Input: part model. Units: mm. Frame: model coordinates. A direction names the side the tool comes from. Give positions to 0.01 mm unless a question says otherwise; leave off trailing zeros. Loops run counter-clockwise (first coordinate to the right, second up) from the corner with the lowest first, then second, coordinate; pieces in that order, holes last. Notation, with made-up numbers: (49, 17.25) - (106, 17.25) arc R17 cw to (106, 29.25) - close; hole circle Ø9 at (51, 61). An arc over 180 degrees is marked (long way). Answer as a JSON object with one key per item and string values.
Autodesk Inventor part; units mm, degrees
ref_plane "Work Plane1" through (31.75, 0, 0) normal (1, 0, 0) x (0, 1, 0)
ref_plane "XZ Plane" through (0, 0, 0) normal (0, 1, 0) x (-1, 0, 0)
ref_plane "XY Plane" through (0, 0, 0) normal (0, 0, 1) x (1, 0, 0)
sketch "Sketch1" plane through (0, 0, 0) normal (0, 1, 0) x (-1, 0, 0)
  circle A0 centre (0, 0) radius 25.4
  circle A1 centre (0, 0) radius 31.75
  dimension "d0" = 50.8
  dimension "d1" = 63.5
extrude "Extrusion1" add sketch "Sketch1" along normal blind 6.35
sketch "Sketch2" plane through (0, 0, 0) normal (0, -1, 0) x (1, 0, 0)
  circle A0 centre (0, 0) radius 25.654
  circle A1 centre (0, 0) radius 31.75
  dimension "d4" = 51.308
extrude "Extrusion2" add sketch "Sketch2" along normal blind 25.4
chamfer "Chamfer1" distance 3.175 angle 45 1 edges at (-25.654, -25.4, 0)
ref_plane "Work Plane1" through (31.75, 0, 0) normal (1, 0, 0) x (0, 1, 0)
sketch "Sketch5" plane through (31.75, 0, 0) normal (1, 0, 0) x (0, 1, 0)
  line L0 (6.35, 31.75) -> (-25.4, 31.75)
  line L1 (-25.4, -31.75) -> (6.35, -31.75)
  line L2 (6.35, 31.75) -> (-25.4, -31.75) construction
  line L3 (-25.4, 31.75) -> (6.35, -31.75) construction
  line L4 (0, 25.654) -> (0, -25.654) construction
  circle A0 centre (-9.525, 25.4) radius 3.35
  circle A1 centre (-9.525, -25.4) radius 3.35
  line L5 (-9.525, 25.4) -> (-9.525, -25.4) construction
  line L6 (6.35, 31.75) -> (6.35, -31.75)
  line L7 (-25.4, 31.75) -> (-25.4, -31.75)
  point P0 (0, 0)
  point P1 (6.35, 0)
  point P2 (-9.525, 0)
  dimension "d27" = 63.5
  dimension "d28" = 50.8
  dimension "d29" = 6.7
extrude "Extrusion4" add sketch "Sketch5" against normal up to surface
mirror "Mirror1" about plane through (0, 0, 0) normal (1, 0, 0) of "Extrusion4"
chamfer "Chamfer3" distance 0.7937 angle 45 7 edges at (0, 6.35, 31.75) (0, 6.35, -31.75) (25.4, 6.35, 0) (31.75, 6.35, 0) (31.75, -25.4, 0) (0, -25.4, -31.75) (0, -25.4, 31.75)
properties part number "WL-002" material "Aluminum 6061"
Item 1: Contact query for flat-ended pins moving along their axis: P1, Ø5.5, axis at y = -9.525, z = -25.4, coming from the -X side; P2, Ø5, axis at x = -8.5, z = 23, coming from the -Y side; P3, Ø6, axis at y = -9.525, z = 25.4, coming from the +X side; P4, Ø12, axis at x = 21, z = 12, coming from the +Y side. Output: stop coordinate, or through.
Geometry check:
{"P1": "stops at x = -22.25", "P2": "stops at y = -23.59", "P3": "stops at x = 22.5", "P4": "stops at y = 6.35"}
Item 2: Cut plane C-C (x = -14.5). Give the number of separate pieces and of enclosed holes in the cut face, then the cut area to 3 significant figures.
Geometry check:
{"separate pieces": "2", "enclosed holes": "2", "area": "660 mm2"}
Item 3: Material intervals for line 1 (Y direction, x = -20, z = -25.4) (3 decimals); line 2 (Z direction, x = 26, y = -9.5); line 3 (Z direction, x = 0, y = -5.25), sorted ascending. Write a range as [from, to].
Geometry check:
{"line 1": "y = [-25.4, -12.875], [-6.175, 6.35]", "line 2": "z = [-31.75, -28.75], [-22.05, 22.05], [28.75, 31.75]", "line 3": "z = [-31.75, -25.65], [25.65, 31.75]"}
Item 4: Mould query, pull axis Y, two halves, no side actions, for faces 5 (the face through (-31.75, -9, 0)), 6 (the face through (0, 6.35, -27)), 7 (the face through (-24.77, -10.25, 28.67)). Classes: released by +Y, released by -Y, zero draft, split by the parting line, or undercut.
Geometry check:
{"face 5": "zero draft", "face 6": "released by +Y", "face 7": "undercut"}
Item 5: Cut plane B-B (y = -15.5). Return loops of the section in (x, z).
Geometry check:
{"outline": "(-31.75, -31.75) - (31.75, -31.75) - (31.75, 31.75) - (-31.75, 31.75) - close; hole circle Ø51.31 at (0, 0)"}
Item 6: Access query for faces 1 (the face through (0, -10, -31.75)), 2 (the face through (-24.77, -9.96, -28.72)), 3 (the face through (24.77, -10.25, -28.67)), 4 (the face through (24.47, -10.96, -7.71)). Directions: +Z, -Z, +X, -X, +Y, -Y. A direction counts if a zero-diameter tool reaches every point of the face in a straight line with its end or side. Return the directions, or none.
Geometry check:
{"face 1": "-Z, +X, -X, +Y, -Y", "face 2": "-X", "face 3": "+X", "face 4": "-Y"}
Item 7: Cut plane A-A (x = 0). Return loops of the section in (y, z) (3 decimals).
Geometry check:
{"outline": "(-25.4, -30.956) - (-24.606, -31.75) - (5.556, -31.75) - (6.35, -30.956) - (6.35, -26.194) - (5.556, -25.4) - (0, -25.4) - (0, -25.654) - (-22.225, -25.654) - (-25.4, -28.829) - close; (-25.4, 28.829) - (-22.225, 25.654) - (0, 25.654) - (0, 25.4) - (5.556, 25.4) - (6.35, 26.194) - (6.35, 30.956) - (5.556, 31.75) - (-24.606, 31.75) - (-25.4, 30.956) - close"}
